from build123d import *

# Parameters (mm, degrees)
SKETCH1_W           = 1193.8
SKETCH1_H           = 386.08
BOSS_EXTRUDE1_DEPTH = 2.667
SKETCH2_W           = 457.2
SKETCH2_H           = 50.8
CUT_EXTRUDE1_DEPTH  = 628.344534119
SKETCH3_W           = 101.6
SKETCH3_H           = 355.6
CUT_EXTRUDE2_DEPTH  = 628.344534119
FILLET1_R           = 4.7625
CUT_EXTRUDE3_DEPTH  = 628.344534119
BOSS_EXTRUDE2_START = -2.667
BOSS_EXTRUDE2_DEPTH = 2.667


with BuildPart() as part:
    # Sketch1 → Boss-Extrude1 (new body)
    with BuildSketch(Plane(origin=(0, 0, 0), x_dir=(1, 0, 0), z_dir=(0, 1, 0))):
        Rectangle(SKETCH1_W, SKETCH1_H)
    extrude(amount=BOSS_EXTRUDE1_DEPTH)

    # Sketch2 → Cut-Extrude1 (cut, through all)
    with BuildSketch(Plane(origin=(0, 2.667, 0), x_dir=(1, 0, 0), z_dir=(0, 1, 0))):
        with Locations((228.6, 0)):
            Rectangle(SKETCH2_W, SKETCH2_H)
        with Locations((-228.6, 0)):
            Rectangle(SKETCH2_W, SKETCH2_H)
    extrude(amount=-CUT_EXTRUDE1_DEPTH, mode=Mode.SUBTRACT)

    # Sketch3 → Cut-Extrude2 (cut, through all)
    with BuildSketch(Plane(origin=(0, 2.667, 0), x_dir=(1, 0, 0), z_dir=(0, 1, 0))):
        Rectangle(SKETCH3_W, SKETCH3_H)
    extrude(amount=-CUT_EXTRUDE2_DEPTH, mode=Mode.SUBTRACT)

    # Fillet1
    fillet1_edges = [part.edges().sort_by_distance(p)[0] for p in [
        (457.2, 1.3335, -25.4),
        (457.2, 1.3335, 25.4),
        (-457.2, 1.3335, 25.4),
        (-457.2, 1.3335, -25.4),
        (-50.8, 1.3335, -25.4),
        (50.8, 1.3335, -25.4),
        (50.8, 1.3335, 25.4),
        (-50.8, 1.3335, 25.4),
        (-50.8, 1.3335, 177.8),
        (50.8, 1.3335, -177.8),
        (50.8, 1.3335, 177.8),
        (-50.8, 1.3335, -177.8),
    ]]
    fillet(fillet1_edges, radius=FILLET1_R)

    # Sketch4 → Cut-Extrude3 (cut, through all)
    with BuildSketch(Plane.XZ):
        with BuildLine():
            Line((-593.892867101, -186.862490674), (-596.9, -76.2))
            Line((-596.9, -76.2), (-596.9, -193.04))
            Line((-596.9, -193.04), (-587.545210292, -193.04))
            ThreePointArc((-587.545210292, -193.04), (-591.973933823, -191.240704109), (-593.892867101, -186.862490674))
        make_face()
        with BuildLine():
            Line((-596.9, 76.2), (-593.892867101, 186.862490674))
            ThreePointArc((-593.892867101, 186.862490674), (-591.973933823, 191.240704109), (-587.545210292, 193.04))
            Line((-587.545210292, 193.04), (-596.9, 193.04))
            Line((-596.9, 193.04), (-596.9, 76.2))
        make_face()
        with BuildLine():
            Line((596.9, 193.04), (587.545210292, 193.04))
            ThreePointArc((587.545210292, 193.04), (591.973933823, 191.240704109), (593.892867101, 186.862490674))
            Line((593.892867101, 186.862490674), (596.9, 76.2))
            Line((596.9, 76.2), (596.9, 193.04))
        make_face()
        with BuildLine():
            ThreePointArc((593.892867101, -186.862490674), (591.973933823, -191.240704109), (587.545210292, -193.04))
            Line((587.545210292, -193.04), (596.9, -193.04))
            Line((596.9, -193.04), (596.9, -76.2))
            Line((596.9, -76.2), (593.892867101, -186.862490674))
        make_face()
    extrude(amount=-CUT_EXTRUDE3_DEPTH, mode=Mode.SUBTRACT)

    # Sketch5 → Boss-Extrude2 (add)
    with BuildSketch(Plane(origin=(0, 2.667, 0), x_dir=(1, 0, 0), z_dir=(0, 1, 0)).offset(BOSS_EXTRUDE2_START)):
        with BuildLine():
            Line((587.545210292, 195.58), (-587.545210292, 195.58))
            ThreePointArc((-587.545210292, 195.58), (-593.745423235, 193.060985753), (-596.431929825, 186.931486944))
            Line((-596.431929825, 186.931486944), (-599.44, 76.234504501))
            Line((-599.44, 76.234504501), (-599.44, -76.234504501))
            Line((-599.44, -76.234504501), (-596.431929825, -186.931486944))
            ThreePointArc((-596.431929825, -186.931486944), (-593.745423235, -193.060985753), (-587.545210292, -195.58))
            Line((-587.545210292, -195.58), (587.545210292, -195.58))
            ThreePointArc((587.545210292, -195.58), (593.745423235, -193.060985753), (596.431929825, -186.931486944))
            Line((596.431929825, -186.931486944), (599.44, -76.234504501))
            Line((599.44, -76.234504501), (599.44, 76.234504501))
            Line((599.44, 76.234504501), (596.431929825, 186.931486944))
            ThreePointArc((596.431929825, 186.931486944), (593.745423235, 193.060985753), (587.545210292, 195.58))
        make_face()
        with BuildLine():
            Line((596.9, 76.2), (593.892867101, 186.862490674))
            ThreePointArc((593.892867101, 186.862490674), (591.973933823, 191.240704109), (587.545210292, 193.04))
            Line((587.545210292, 193.04), (-587.545210292, 193.04))
            ThreePointArc((-587.545210292, 193.04), (-591.973933823, 191.240704109), (-593.892867101, 186.862490674))
            Line((-593.892867101, 186.862490674), (-596.9, 76.2))
            Line((-596.9, 76.2), (-596.9, -76.2))
            Line((-596.9, -76.2), (-593.892867101, -186.862490674))
            ThreePointArc((-593.892867101, -186.862490674), (-591.973933823, -191.240704109), (-587.545210292, -193.04))
            Line((-587.545210292, -193.04), (587.545210292, -193.04))
            ThreePointArc((587.545210292, -193.04), (591.973933823, -191.240704109), (593.892867101, -186.862490674))
            Line((593.892867101, -186.862490674), (596.9, -76.2))
            Line((596.9, -76.2), (596.9, 76.2))
        make_face(mode=Mode.SUBTRACT)
    extrude(amount=BOSS_EXTRUDE2_DEPTH)


solid = part.part
Geometry check sheet. Reference: the model listing, model coordinates, mm. Coordinates: 2 decimals unless noted, no trailing zeros. Order: outer loops, then holes, each group sorted by start corner. A loop starts at its lowest first (then second) coordinate and runs counter-clockwise, first axis right, second up. Notation, with made-up numbers: (82, 69.5) - (139, 69.5) arc R20 cw to (139, 100.5) - close; hole circle Ø11 at (-26.5, 9.5). An arc over 180 degrees is marked (long way). One line per item, written item: value.
(1) Sectioned sample at A-A (x = 3.5). Enter the section's corners in (y, z), and give its area (3 significant figures).
Data:
outline: (0, -195.58) - (2.67, -195.58) - (2.67, -177.8) - (0, -177.8) - close; (0, 177.8) - (2.67, 177.8) - (2.67, 195.58) - (0, 195.58) - close
area: 94.8 mm^2
(2) Sectioned sample at B-B (z = 1.5). Enter the section's corners in (x, y), and give its area (3 significant figures).
Data:
outline: (-599.44, 0) - (-457.2, 0) - (-457.2, 2.67) - (-599.44, 2.67) - close; (457.2, 0) - (599.44, 0) - (599.44, 2.67) - (457.2, 2.67) - close
area: 759 mm^2
(3) Depth check by flat-ended pin: pin 1 Ø1.3 at (y, z) = (1, -132) entering from +X; pin 2 Ø1.5 at (y, z) = (1.5, 109.5) entering from +X; pin 3 Ø1.3 at (y, z) = (1.5, 84.5) entering from +X. Enter the tip coordinate at first touch or a pass-through.
Data:
pin 1: stops at x = 597.94
pin 2: stops at x = 598.56
pin 3: stops at x = 599.23
(4) Thickness scan on probe 1 along X at (y, z) = (0.75, -60.5); probe 2 along X at (y, z) = (1.5, 3); probe 3 along Z at (x, y) = (115, 1.35). Record the ranges inside material, lowest first. Write a range as from..to.
Data:
probe 1: x = -599.44..-50.8, 50.8..599.44
probe 2: x = -599.44..-457.2, 457.2..599.44
probe 3: z = -195.58..-25.4, 25.4..195.58
